The figure shows three views and two pictorial views of one solid part (mm, origin at its lowest corner). Answer the questions. A direction names the side the tool comes from. Round coordinates to 2 decimals unless told otherwise and drop trailing zeros. Order: outer loops, then holes, each group sorted by start corner. A loop starts at its lowest first (then second) coordinate and runs counter-clockwise, first axis right, second up. Notation, with made-up numbers: (-24, 9) - (21, 9) arc R37 cw to (21, 47) - close; hole circle Ø9 at (59, 70.5). An arc over 180 degrees is marked (long way). One line per item, written item: value. Start each with the question number.
1. Section D-D, the plane y = 9.5 is taken. Give the vertices of the cut face in (x, z), then the cut area to 3 significant figures.
2. For a pull along Y with two mould halves and no side action, classify the marked faces 1, 2 and 3 as released by +Y, released by -Y, zero draft, split by the parting line, or undercut.
3. A tool of negligible diameter and unlimited length cuts with its end or side. For the marked faces 4 and 5, from which of +Z, -Z, +X, -X, +Y, -Y can it reach the whole face along a straight path? Write none if from no direction.
4. Flat-ended cylindrical pins translate along their axes: P1, Ø1, axis at x = 5, z = 3, coming from the +Y side; P2, Ø6.5, axis at x = 5.5, y = 6, coming from the -Z side; P3, Ø3, axis at y = 5.5, z = 5.5, coming from the -X side; P4, Ø1, axis at x = 10, z = 3.5, coming from the +Y side. Find the tip coordinate at first contact, or state that the pin passes through.
5. Straight lines are drawn through the part: line 1 (Z direction, x = 10.25, y = 1.5); line 2 (Y direction, x = 6.5, z = 6.75); line 3 (Y direction, x = 7.75, z = 3.75). For each, find the intervals that lie inside material, in ascending order.
6. Section A-A, the plane y = 6.5 is taken. Give the vertices of the cut face in (x, z).
7. Section C-C, the plane z = 6 is taken. Give the vertices of the cut face in (x, y), then the cut area to 3 significant figures.
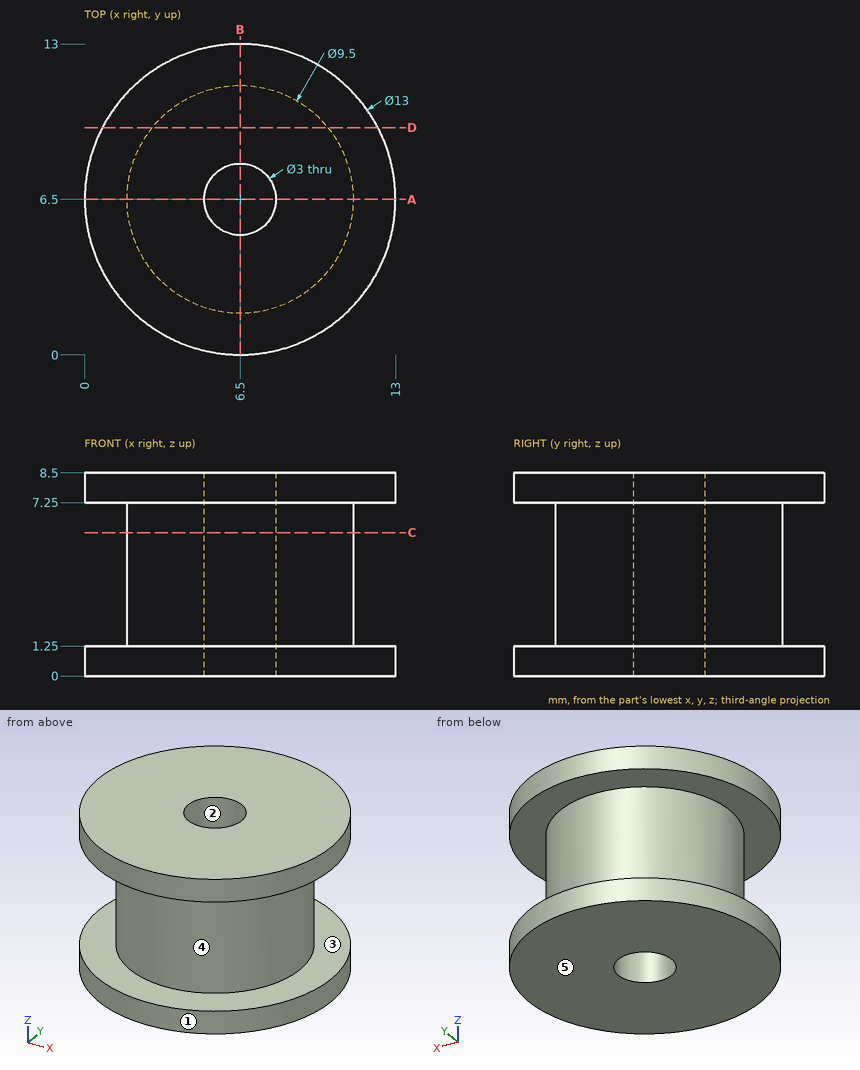
Answer list:
1. outline: (0.73, 0) - (12.27, 0) - (12.27, 1.25) - (10.18, 1.25) - (10.18, 7.25) - (12.27, 7.25) - (12.27, 8.5) - (0.73, 8.5) - (0.73, 7.25) - (2.82, 7.25) - (2.82, 1.25) - (0.73, 1.25) - close
1. area: 73.0 mm²
2. face 1: split by the parting line
2. face 2: undercut
2. face 3: zero draft
3. face 4: none
3. face 5: -Z, +X, -X, +Y, -Y
4. P1: stops at y = 11.14
4. P2: stops at z = 0
4. P3: stops at x = 1.75
4. P4: stops at y = 10.18
5. line 1: z = 0 to 1.25, 7.25 to 8.5
5. line 2: y = 1.75 to 5, 8 to 11.25
5. line 3: y = 1.92 to 5.67, 7.33 to 11.08
6. outline: (0, 0) - (5, 0) - (5, 8.5) - (0, 8.5) - (0, 7.25) - (1.75, 7.25) - (1.75, 1.25) - (0, 1.25) - close; (8, 0) - (13, 0) - (13, 1.25) - (11.25, 1.25) - (11.25, 7.25) - (13, 7.25) - (13, 8.5) - (8, 8.5) - close
7. outline: circle Ø9.5 at (6.5, 6.5); hole circle Ø3 at (6.5, 6.5)
7. area: 63.8 mm²
